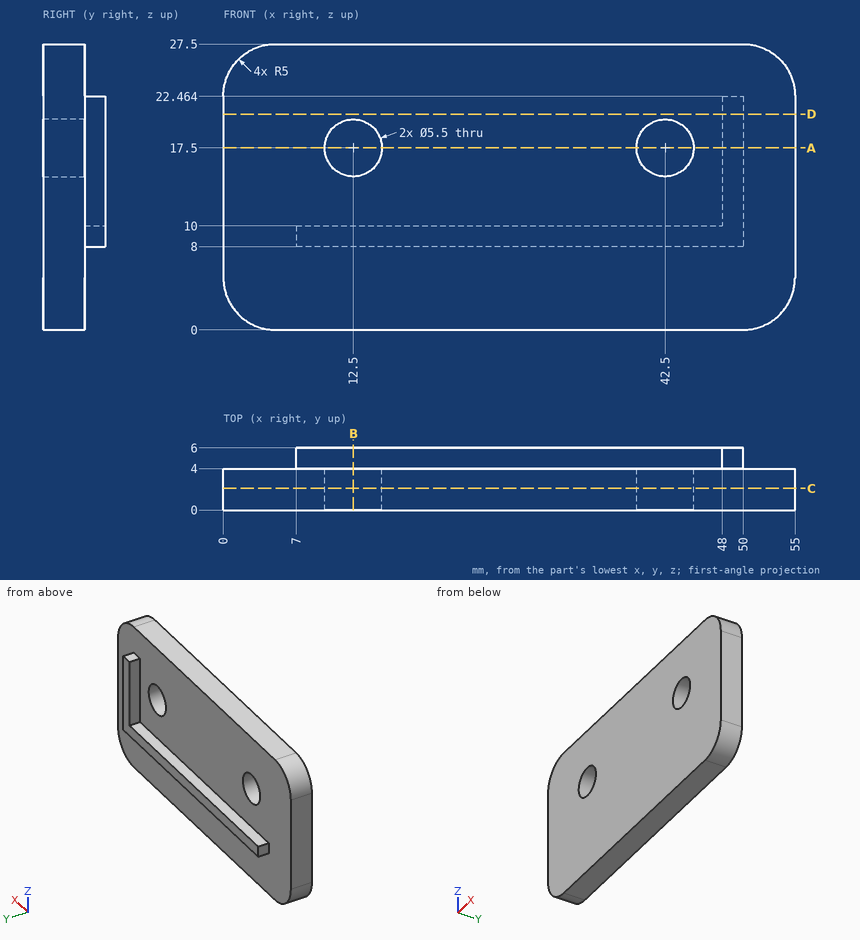
Here's the drawing with two shaded views (mm, measured from the low corner). I have some questions. Coordinates: 2 decimals unless noted, no trailing zeros. Write each loop counter-clockwise with the first axis right and the second up, starting at its lowest first coordinate (ties: lowest second). Pieces come first, ordered by that corner, then holes. Notation, with made-up numbers: M -37,52 L 8,52 A21 cw 8,85 Z; hole C 40,23 d8. An arc over 180 degrees is marked long. Use one line per item in the form item = value.
Q1. If we section it at A-A (z = 17.5): Write out the boundary of the cut face in (x, y).
Model answer:
outline = M 0,0 L 9.75,0 L 9.75,4 L 0,4 Z; M 15.25,0 L 39.75,0 L 39.75,4 L 15.25,4 Z; M 45.25,0 L 55,0 L 55,4 L 50,4 L 50,6 L 48,6 L 48,4 L 45.25,4 Z
Q2. If we section it at B-B (x = 12.5): Write out the boundary of the cut face in (y, z).
Model answer:
outline = M 0,0 L 4,0 L 4,8 L 6,8 L 6,10 L 4,10 L 4,14.75 L 0,14.75 Z; M 0,20.25 L 4,20.25 L 4,27.5 L 0,27.5 Z
Q3. For P1, Ø1.5, axis at y = 4.5, z = 24, coming from the +X side; P2, Ø5, axis at x = 12.5, z = 17.5, coming from the +Y side; P3, Ø1.6, axis at y = 5, z = 17, coming from the -X side; P4, Ø0.6, axis at y = 4.5, z = 18, coming from the +X side, each with a flat end and sliding along its axis, tell me the tip position at first contact or that it passes through.
Model answer:
P1 = 54.91
P2 = through
P3 = 48
P4 = 50
Q4. I need wall thicknesses on line 1 along X through (y, z) = (2.75, 17.5); line 2 along X through (y, z) = (1.15, 18.5); line 3 along Z through (x, y) = (12.5, 2.6). Which ranges of each line are inside material? Lowest first, please. Write a range as from..to.
Model answer:
line_1 = 0..9.75, 15.25..39.75, 45.25..55
line_2 = 0..9.94, 15.06..39.94, 45.06..55
line_3 = 0..14.75, 20.25..27.5
Q5. If we section it at C-C (y = 2.1): Write out the boundary of the cut face in (x, z).
Model answer:
outline = M 0,5 A5 ccw 5,0 L 50,0 A5 ccw 55,5 L 55,22.5 A5 ccw 50,27.5 L 5,27.5 A5 ccw 0,22.5 Z; hole C 12.5,17.5 d5.5; hole C 42.5,17.5 d5.5
Q6. If we section it at D-D (z = 20.75): Write out the boundary of the cut face in (x, y).
Model answer:
outline = M 0,0 L 55,0 L 55,4 L 50,4 L 50,6 L 48,6 L 48,4 L 0,4 Z
